The figure shows three views and two pictorial views of one solid part (mm, origin at its lowest corner). Answer the questions. Give positions to 0.01 mm unless a question says otherwise; leave off trailing zeros. Order: outer loops, then holes, each group sorted by start corner. A loop starts at its lowest first (then second) coordinate and runs counter-clockwise, first axis right, second up. Notation, with made-up numbers: (38, 67) - (55, 67) arc R25 ccw to (55, 95) - close; hole circle Ø6 at (49, 23.25). An arc over 180 degrees is marked (long way). Return JSON: item names as keys, results as strings. Group by question number.
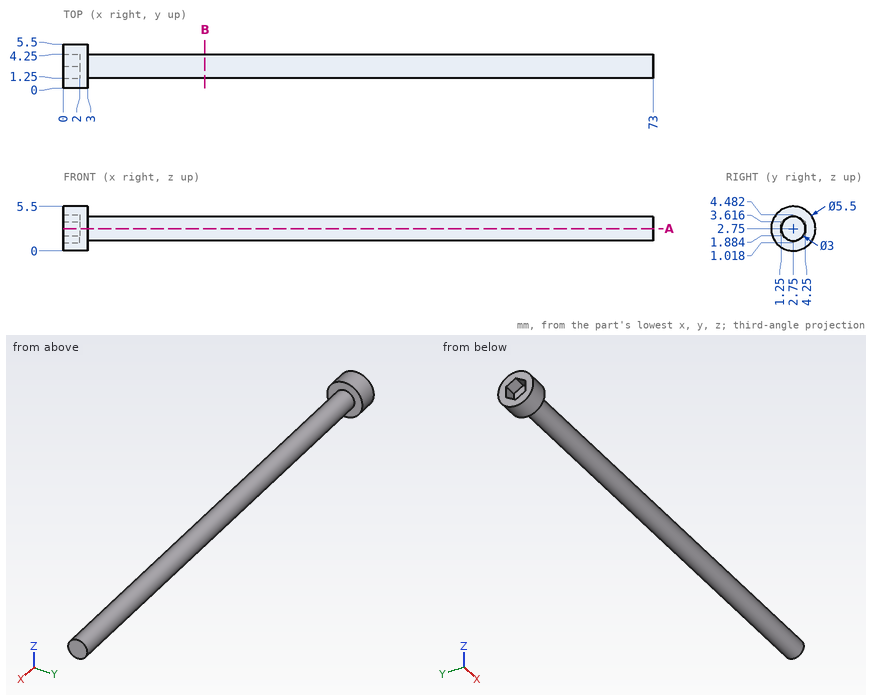
1. Consider probe 1 along X at (y, z) = (2.15, 3.3); probe 2 along Y at (x, z) = (53, 2.6); probe 3 along X at (y, z) = (3.2, 0.4). Determine where each line is inside the solid, lowest interval first. Write a range as from..to.
2. The part is cut by section A-A (z = 2.75). Give the vertices of the cut face in (x, y).
3. Each of these flat-tipped pins is pushed along its axis until it touches: pin 1 (1.5 mm diameter, centred on x = 21, z = 1, fed in from +Y); pin 2 (3 mm diameter, centred on x = 36.5, z = 2.5, fed in from +Y); pin 3 (2 mm diameter, centred on x = 18, y = 0.5, fed in from -Z). Where does it stop, or does it pass through?
4. The part is cut by section B-B (x = 17.5). Give the vertices of the cut face in (y, z), and give its area (3 significant figures).
Answers:
{
 "1": {"probe 1": "x = 2..73", "probe 2": "y = 1.26..4.24", "probe 3": "x = 0..3"},
 "2": {"outline": "(0, 0) - (3, 0) - (3, 1.25) - (73, 1.25) - (73, 4.25) - (3, 4.25) - (3, 5.5) - (0, 5.5) - (0, 4.25) - (2, 4.25) - (2, 1.25) - (0, 1.25) - close"},
 "3": {"pin 1": "stops at y = 3.87", "pin 2": "stops at y = 4.25", "pin 3": "stops at z = 1.92"},
 "4": {"outline": "circle Ø3 at (2.75, 2.75)", "area": "7.07 mm^2"}
}
